For this review, take the finished solid that the model builds, in its own axes (mm). A direction names the side the tool comes from. Give positions to 0.01 mm unless a question says otherwise; leave off trailing zeros. Order: outer loops, then holes, each group sorted by start corner. A loop starts at its lowest first (then second) coordinate and runs counter-clockwise, first axis right, second up. Notation, with made-up numbers: (-8.75, 67) - (26.25, 67) arc R24 ccw to (26.25, 99) - close; hole circle Ø9 at (-5, 37.5). An arc over 180 degrees is marked (long way). Use a Markdown table: item, result. Add a question column.
1) We need section C-C on x = -25. Write out the cut boundary in (y, z).
2) We need section D-D on x = 10. Write out the cut boundary in (y, z).
3) Machinability: for faces 1 (the face through (-25, 10.16, 0)), 2 (the face through (-30, 0, 1.588)), 3 (the face through (-1, 0, -1.588)), 4 (the face through (-26.12, -8.87, 0.05)), which of the approach directions +Z, -Z, +X, -X, +Y, -Y give a long, thin tool a straight path to every point of the face, cutting with its end or side? Answer none if there is none.
4) Wall thickness on L1, parallel to Z at x = -3.5, y = 11.5; L2, parallel to Y at x = -29, z = 0; L3, parallel to Y at x = -24, z = -0.75: over which ranges is each line inside the solid? List them lowest first.
5) Clearance check with flat-ended pins moving along their axes: P1, Ø1.8, axis at x = -25, z = 0.5, coming from the -Y side; P2, Ø3.5, axis at x = -30, z = -0.5, coming from the +Y side; P3, Ø1.5, axis at x = -14.5, y = -10, coming from the -Z side. State where each tip first meets the part, or that it passes through.
6) Mouldability with a two-part tool opening along X and no side actions: class faces 5 (the face through (-27.478, 0.107, -1.72)), 6 (the face through (-30, 6.35, 0)), 7 (the face through (-23.92, 8.87, 0.05)) as released by +X, released by -X, zero draft, split by the parting line, or undercut.
7) We need section A-A on y = -4.5. Write out the cut boundary in (x, z).
8) We need section B-B on z = 0. Write out the cut boundary in (x, y), then the cut area to 3 significant figures.
```python
from build123d import *

# Parameters (mm, degrees)
F2_DEPTH = 1.5875
F4_R     = 1.1
F5_DEPTH = 2.54
F3_R     = 1.1
F6_DEPTH = 2.54


with BuildPart() as f1:
    # F0 (on Top) → F1 (revolve)
    with BuildSketch(Plane.XY):
        Polygon((-25.0192951104, 6.35), (-25.0192951104, 0), (-25.0192951104, -6.35), (-22.0192951104, -6.35), (-22.0192951104, 6.35), align=None)
        Polygon((-25.0192951104, 7.62), (-25.0192951104, 6.35), (-22.0192951104, 7.25), (-22.0192951104, 7.62), align=None)
        Polygon((-22.0192951104, -7.25), (-25.0192951104, -6.35), (-25.0192951104, -7.62), (-22.0192951104, -7.62), align=None)
        Polygon((-22.0192951104, -6.35), (-25.0192951104, -6.35), (-22.0192951104, -7.25), align=None)
        Polygon((-22.0192951104, 7.25), (-25.0192951104, 6.35), (-22.0192951104, 6.35), align=None)
    revolve(axis=Axis((-25.0192951104, 3.175, 0), (0, 1, 0)))

    # F0 (on Top) → F2 (join, symmetric)
    with BuildSketch(Plane.XY):
        Polygon((-25.0192951104, 6.35), (-25.0192951104, 0), (-25.0192951104, -6.35), (-22.0192951104, -6.35), (-22.0192951104, 6.35), align=None)
        Polygon((-25.0192951104, -6.35), (-25.0192951104, 0), (-25.0192951104, 6.35), (-32.6392951104, 6.35), (-32.6392951104, -6.35), align=None)
        Polygon((-22.0192951104, -6.35), (-25.0192951104, -6.35), (-22.0192951104, -7.25), align=None)
        Polygon((-22.0192951104, -7.25), (-25.0192951104, -6.35), (-25.0192951104, -7.62), (-22.0192951104, -7.62), align=None)
        Polygon((-25.0192951104, 7.62), (-25.0192951104, 6.35), (-22.0192951104, 7.25), (-22.0192951104, 7.62), align=None)
        Polygon((-22.0192951104, 7.25), (-25.0192951104, 6.35), (-22.0192951104, 6.35), align=None)
        Polygon((-22.0192951104, -6.35), (-22.0192951104, -7.25), (13.0807048896, -17.78), (13.0807048896, 0), (13.0807048896, 17.78), (-22.0192951104, 7.25), (-22.0192951104, 6.35), align=None)
    extrude(amount=F2_DEPTH, both=True)

    # F4 (on face) → F5 (join)
    with BuildSketch(Plane(origin=(0, 7.62, 0), x_dir=(-1, 0, 0), z_dir=(0, 1, 0))):
        with Locations((25.0192951104, 0)):
            Circle(F4_R)
    extrude(amount=F5_DEPTH)

    # F3 (on face) → F6 (join)
    with BuildSketch(Plane.XZ.offset(7.62)):
        with Locations((-25.0192951104, 0)):
            Circle(F3_R)
    extrude(amount=F6_DEPTH)


solid = f1.part
```
Checked values:
| question | item | result |
|---|---|---|
| 1 | outline | (-10.16, -1.1) - (-7.62, -1.1) - (-7.62, -3) - (7.62, -3) - (7.62, -1.1) - (10.16, -1.1) - (10.16, 1.1) - (7.62, 1.1) - (7.62, 3) - (-7.62, 3) - (-7.62, 1.1) - (-10.16, 1.1) - close |
| 2 | outline | (-16.86, -1.59) - (16.86, -1.59) - (16.86, 1.59) - (-16.86, 1.59) - close |
| 3 | face 1 | +Z, -Z, -X, +Y |
| 3 | face 2 | +Z, -X, +Y, -Y |
| 3 | face 3 | -Z, +X, +Y, -Y |
| 3 | face 4 | -Y |
| 4 | L1 | -1.59 to 1.59 |
| 4 | L2 | -6.35 to 6.35 |
| 4 | L3 | -7.62 to 7.62 |
| 5 | P1 | y = -10.16 |
| 5 | P2 | y = 6.35 |
| 5 | P3 | z = -1.59 |
| 6 | face 5 | split by the parting line |
| 6 | face 6 | zero draft |
| 6 | face 7 | undercut |
| 7 | outline | (-32.64, -1.59) - (-27.56, -1.59) arc R3 ccw to (-22.47, -1.59) - (13.08, -1.59) - (13.08, 1.59) - (-22.47, 1.59) arc R3 ccw to (-27.56, 1.59) - (-32.64, 1.59) - close |
| 8 | outline | (-32.64, -6.35) - (-28.02, -6.35) - (-28.02, -7.62) - (-26.12, -7.62) - (-26.12, -10.16) - (-23.92, -10.16) - (-23.92, -7.62) - (-22.02, -7.62) - (-22.02, -7.25) - (13.08, -17.78) - (13.08, 17.78) - (-22.02, 7.25) - (-22.02, 7.62) - (-23.92, 7.62) - (-23.92, 10.16) - (-26.12, 10.16) - (-26.12, 7.62) - (-28.02, 7.62) - (-28.02, 6.35) - (-32.64, 6.35) - close |
| 8 | area | 1,040 mm² |
